The listing builds one solid part. Answer for the finished solid, in the listing's coordinates (mm). Face numbers are marked on the shaded views. Coordinates: 2 decimals unless noted, no trailing zeros. Loops run counter-clockwise (first coordinate to the right, second up) from the corner with the lowest first, then second, coordinate; pieces in that order, holes last. Notation, with made-up numbers: (76.5, 47.25) -> (134.5, 47.25) arc R5 cw to (134.5, 51.25) -> close; hole circle Ø6 at (-7.75, -25). An arc over 180 degrees is marked (long way). Answer in a Markdown table with one row per item.
```python
from build123d import *

# Parameters (mm, degrees)
F0_R     = 1.5
F1_DEPTH = 48
F2_W     = 5
F2_H     = 12
F3_DEPTH = 5


with BuildPart() as f1:
    # F0 (on Front) → F1 (new body)
    with BuildSketch(Plane.XZ):
        with BuildLine():
            Line((-1.5, 2), (-15, 2))
            Line((-15, 2), (-15, 0))
            Line((-15, 0), (-2.5, 0))
            ThreePointArc((-2.5, 0), (2.2360679775, -1.1180339887), (-1.5, 2))
        make_face()
        Circle(F0_R, mode=Mode.SUBTRACT)
    extrude(amount=F1_DEPTH)

    # F2 (on face) → F3 (cut, symmetric)
    with BuildSketch(Plane(origin=(0, 0, 0), x_dir=(1, 0, 0), z_dir=(0, 0, -1))):
        with Locations((0, 6)):
            Rectangle(F2_W, F2_H)
        with Locations((0, 30)):
            Rectangle(F2_W, F2_H)
    extrude(amount=F3_DEPTH, both=True, mode=Mode.SUBTRACT)


solid = f1.part
```
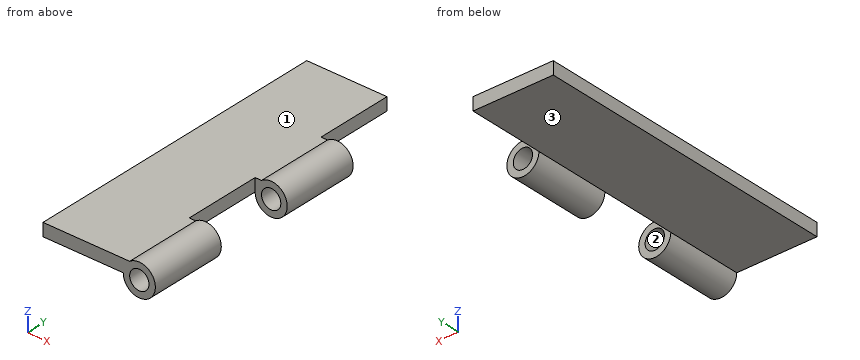
Item 1: Flat-ended cylindrical pins translate along their axes: pin 1 Ø1.5 at (x, y) = (-2.5, -7) entering from -Z; pin 2 Ø1.8 at (x, z) = (0, 0) entering from -Y; pin 3 Ø1.6 at (y, z) = (-33, 1) entering from +X. Find the tip coordinate at first contact, or state that the pin passes through.
Findings below:
| item | result |
|---|---|
| pin 1 | stops at z = 0 |
| pin 2 | passes through |
| pin 3 | stops at x = -2.5 |
Item 2: A cutting plane is placed at A-A, the plane x = 0. Determine the outline of the cut face in (y, z).
Findings below:
| item | result |
|---|---|
| outline | (-48, -2.5) -> (-36, -2.5) -> (-36, -1.5) -> (-48, -1.5) -> close; (-48, 1.5) -> (-36, 1.5) -> (-36, 2.5) -> (-48, 2.5) -> close; (-24, -2.5) -> (-12, -2.5) -> (-12, -1.5) -> (-24, -1.5) -> close; (-24, 1.5) -> (-12, 1.5) -> (-12, 2.5) -> (-24, 2.5) -> close |
Item 3: Determine the mould class of the marked faces 1, 2 and 3 for opening direction Z: +Z half, -Z half, draft (parallel to the pull), parting line (faces both ways), or undercut.
Findings below:
| item | result |
|---|---|
| face 1 | +Z half |
| face 2 | undercut |
| face 3 | -Z half |
Item 4: Find the intervals of material crossed by probe 1 along Z at (x, y) = (0, -42); probe 2 along Y at (x, z) = (-1.75, -0.45); probe 3 along Z at (x, y) = (-12.75, -8), in increasing order.
Findings below:
| item | result |
|---|---|
| probe 1 | z = -2.5 to -1.5, 1.5 to 2.5 |
| probe 2 | y = -48 to -36, -24 to -12 |
| probe 3 | z = 0 to 2 |
Item 5: A cutting plane is placed at B-B, the plane y = -38.5. Determine the outline of the cut face in (x, z), plus the area to 3 significant figures.
Findings below:
| item | result |
|---|---|
| outline | (-15, 0) -> (-2.5, 0) arc R2.5 ccw (long way) to (-1.5, 2) -> (-15, 2) -> close; hole circle Ø3 at (0, 0) |
| area | 38.2 mm2 |
Item 6: A cutting plane is placed at D-D, the plane x = -13. Determine the outline of the cut face in (y, z).
Findings below:
| item | result |
|---|---|
| outline | (-48, 0) -> (0, 0) -> (0, 2) -> (-48, 2) -> close |
Item 7: A cutting plane is placed at C-C, the plane y = -28.5. Determine the outline of the cut face in (x, z), plus the area to 3 significant figures.
Findings below:
| item | result |
|---|---|
| outline | (-15, 0) -> (-2.5, 0) -> (-2.5, 2) -> (-15, 2) -> close |
| area | 25.0 mm2 |
